Autodesk Fusion 360 part; units mm, degrees
sketch "Sketch1" plane through (0, 0, 0) normal (0, 0, 1) x (1, 0, 0)
  line L0 (69.2401, 97.5535) -> (12.2401, 97.5535)
  line L1 (12.2401, 97.5535) -> (12.2401, 48.4535)
  line L2 (52.8401, 84.1535) -> (28.6401, 84.1535)
  line L3 (59.3712, 82.4035) -> (64.1343, 79.6535)
  line L4 (64.1343, 79.6535) -> (69.2401, 79.6535)
  line L5 (69.2401, 79.6535) -> (69.2401, 97.5535)
  line L6 (22.109, 82.4035) -> (14.2401, 77.8603)
  line L7 (14.2401, 77.8603) -> (14.2401, 61.3991)
  line L8 (14.2401, 61.3991) -> (22.3734, 55.0972)
  line L9 (28.5401, 52.1228) -> (28.5401, 48.4535)
  line L10 (28.5401, 48.4535) -> (12.2401, 48.4535)
  arc A0 (59.3712, 82.4035) -> (52.8401, 84.1535) centre (56.3401, 84.1535) ccw
  arc A1 (28.6401, 84.1535) -> (22.109, 82.4035) centre (25.1401, 84.1535) ccw
  arc A2 (22.3734, 55.0972) -> (28.5401, 52.1228) centre (25.1401, 52.9535) ccw
  line L11 (14.2401, 50.4535) -> (14.2401, 58.869)
  line L12 (14.2401, 58.869) -> (19.6401, 54.6849)
  line L13 (19.6401, 54.6849) -> (14.2401, 50.4535)
  line L14 (14.2401, 86.1535) -> (22.9682, 95.5535)
  line L15 (22.9682, 95.5535) -> (14.2401, 95.5535)
  line L16 (14.2401, 95.5535) -> (14.2401, 86.1535)
  line L17 (26.3674, 95.5535) -> (32.3674, 86.1535)
  line L18 (32.3674, 86.1535) -> (38.3674, 95.5535)
  line L19 (38.3674, 95.5535) -> (26.3674, 95.5535)
  line L20 (49.1128, 86.1535) -> (55.1128, 95.5535)
  line L21 (55.1128, 95.5535) -> (43.1128, 95.5535)
  line L22 (43.1128, 95.5535) -> (49.1128, 86.1535)
  line L23 (34.7401, 86.1535) -> (46.7401, 86.1535)
  line L24 (46.7401, 86.1535) -> (40.7401, 95.5535)
  line L25 (40.7401, 95.5535) -> (34.7401, 86.1535)
  dimension "d1" = 7
  dimension "d2" = 7
  dimension "d3" = 31.2
  dimension "d10" = 7
  dimension "d11" = 150
  dimension "d12" = 150
  dimension "d13" = 127.769
  dimension "d14" = 12.9
  dimension "d15" = 12.9
  dimension "d16" = 31.2
  dimension "d17" = 4.5
  dimension "d18" = 13.4
  dimension "d19" = 12.9
  dimension "d21" = 4.5
  dimension "d23" = 2
  dimension "d24" = 5.5
  dimension "d25" = 2
  dimension "d26" = 2
  dimension "d27" = 2
  dimension "d35" = 2
  dimension "d36" = 2
  dimension "d37" = 2
  dimension "d38" = 2
  dimension "d39" = 2
  dimension "d40" = 2
  dimension "d41" = 2
  dimension "d42" = 2
  dimension "d43" = 2
  dimension "d44" = 2
  dimension "d45" = 12
  dimension "d46" = 15.6
  dimension "d47" = 2
  dimension "d74" = 90
  dimension "d77" = 3.4
extrude "Extrude1" add sketch "Sketch1" along normal blind 12.5
sketch "Sketch2" plane through (0, 97.5535, 0) normal (0, 1, 0) x (-1, 0, 0)
  line L0 (-69.2401, 0) -> (-12.2401, 0)
  line L1 (-12.2401, 0) -> (-12.2401, 12.5)
  line L2 (-12.2401, 12.5) -> (-69.2401, 12.5)
  line L3 (-69.2401, 12.5) -> (-69.2401, 0)
  point P0 (-60.2401, 4.5)
  dimension "d30" = 9
  dimension "d31" = 8
hole "Hole1" at (60.2401, 97.5535, 4.5) direction (0, -1, 0) diameter 5 depth 10 tip angle 118
fillet "Fillet2" radius 1 15 edges at (55.1128, 95.5535, 6.25) (43.1128, 95.5535, 6.25) (49.1128, 86.1535, 6.25) (46.7401, 86.1535, 6.25) (40.7401, 95.5535, 6.25) (34.7401, 86.1535, 6.25) (38.3674, 95.5535, 6.25) (32.3674, 86.1535, 6.25) (26.3674, 95.5535, 6.25) (22.9682, 95.5535, 6.25) (14.2401, 86.1535, 6.25) (14.2401, 95.5535, 6.25) (19.6401, 54.6849, 6.25) (14.2401, 58.869, 6.25) (14.2401, 50.4535, 6.25)
sketch "Sketch3" plane through (0, 0, 0) normal (0, 0, -1) x (1, 0, 0)
  line L0 (69.2401, -79.6535) -> (64.1343, -79.6535)
  line L1 (64.1343, -79.6535) -> (59.3712, -82.4035)
  arc A0 (52.8401, -84.1535) -> (59.3712, -82.4035) centre (56.3401, -84.1535) ccw
  line L2 (52.8401, -84.1535) -> (28.6401, -84.1535)
  arc A1 (22.109, -82.4035) -> (28.6401, -84.1535) centre (25.1401, -84.1535) ccw
  line L3 (22.109, -82.4035) -> (14.2401, -77.8603)
  line L4 (14.2401, -77.8603) -> (14.2401, -61.3991)
  line L5 (14.2401, -61.3991) -> (22.3734, -55.0972)
  arc A2 (28.5401, -52.1228) -> (22.3734, -55.0972) centre (25.1401, -52.9535) ccw
  line L6 (28.5401, -52.1228) -> (28.5401, -48.4535)
  line L7 (28.5401, -48.4535) -> (12.2401, -48.4535)
  line L8 (12.2401, -48.4535) -> (12.2401, -97.5535)
  line L9 (12.2401, -97.5535) -> (69.2401, -97.5535)
  line L10 (69.2401, -97.5535) -> (69.2401, -79.6535)
  arc A3 (27.3491, -94.0154) -> (28.1921, -95.5535) centre (28.1921, -94.5535) ccw
  line L11 (27.3491, -94.0154) -> (31.5245, -87.474)
  arc A4 (33.2103, -87.474) -> (31.5245, -87.474) centre (32.3674, -88.0121) ccw
  line L12 (33.2103, -87.474) -> (37.3857, -94.0154)
  arc A5 (36.5428, -95.5535) -> (37.3857, -94.0154) centre (36.5428, -94.5535) ccw
  line L13 (36.5428, -95.5535) -> (28.1921, -95.5535)
  arc A6 (14.2401, -56.8291) -> (15.8526, -57.6196) centre (15.2401, -56.8291) ccw
  line L14 (14.2401, -56.8291) -> (14.2401, -52.5075)
  arc A7 (15.8569, -51.7204) -> (14.2401, -52.5075) centre (15.2401, -52.5075) ccw
  line L15 (15.8569, -51.7204) -> (18.6299, -53.8933)
  arc A8 (18.6256, -55.4709) -> (18.6299, -53.8933) centre (18.0131, -54.6805) ccw
  line L16 (18.6256, -55.4709) -> (15.8526, -57.6196)
  arc A9 (15.9729, -88.0197) -> (14.2401, -88.7001) centre (15.2401, -88.7001) ccw
  line L17 (15.9729, -88.0197) -> (21.4079, -93.873)
  arc A10 (20.6751, -95.5535) -> (21.4079, -93.873) centre (20.6751, -94.5535) ccw
  line L18 (20.6751, -95.5535) -> (15.2401, -95.5535)
  arc A11 (14.2401, -94.5535) -> (15.2401, -95.5535) centre (15.2401, -94.5535) ccw
  line L19 (14.2401, -94.5535) -> (14.2401, -88.7001)
  arc A12 (49.9557, -87.474) -> (48.2699, -87.474) centre (49.1128, -88.0121) ccw
  line L20 (49.9557, -87.474) -> (54.1311, -94.0154)
  arc A13 (53.2882, -95.5535) -> (54.1311, -94.0154) centre (53.2882, -94.5535) ccw
  line L21 (53.2882, -95.5535) -> (44.9375, -95.5535)
  arc A14 (44.0945, -94.0154) -> (44.9375, -95.5535) centre (44.9375, -94.5535) ccw
  line L22 (44.0945, -94.0154) -> (48.2699, -87.474)
  arc A15 (36.5648, -86.1535) -> (35.7218, -87.6915) centre (36.5648, -87.1535) ccw
  line L23 (36.5648, -86.1535) -> (44.9155, -86.1535)
  arc A16 (45.7584, -87.6915) -> (44.9155, -86.1535) centre (44.9155, -87.1535) ccw
  line L24 (45.7584, -87.6915) -> (41.583, -94.2329)
  arc A17 (39.8972, -94.2329) -> (41.583, -94.2329) centre (40.7401, -93.6948) ccw
  line L25 (39.8972, -94.2329) -> (35.7218, -87.6915)
  line L26 (12.2401, -48.4535) -> (14.2401, -48.4535)
  line L27 (12.2401, -48.4535) -> (12.2401, -97.5535)
  line L28 (12.2401, -97.5535) -> (14.2401, -97.5535)
  line L29 (14.2401, -97.5535) -> (14.2401, -48.4535)
  dimension "d51" = 2
  dimension "d52" = 2
extrude "Extrude2" add sketch "Sketch3" along normal blind 7.5 contours L4 L7 L8 L9 L14 L19 L26 L27 L28 L29
sketch "Sketch4" plane through (12.2401, 0, 0) normal (-1, 0, 0) x (0, -1, 0)
  line L0 (-48.4535, -7.5) -> (-48.4535, 12.5)
  line L1 (-48.4535, 12.5) -> (-97.5535, 12.5)
  line L2 (-97.5535, 12.5) -> (-97.5535, -7.5)
  line L3 (-97.5535, -7.5) -> (-48.4535, -7.5)
  line L4 (-93.5535, -1.3) -> (-73.5535, -1.3)
  arc A0 (-73.5535, -3.7) -> (-73.5535, -1.3) centre (-73.5535, -2.5) ccw
  line L5 (-73.5535, -3.7) -> (-93.5535, -3.7)
  arc A1 (-93.5535, -1.3) -> (-93.5535, -3.7) centre (-93.5535, -2.5) ccw
  arc A2 (-93.5535, 8.8) -> (-93.5535, 6.4) centre (-93.5535, 7.6) ccw
  arc A3 (-73.5535, 6.4) -> (-73.5535, 8.8) centre (-73.5535, 7.6) ccw
  line L6 (-73.5535, 6.4) -> (-93.5535, 6.4)
  line L7 (-93.5535, 8.8) -> (-73.5535, 8.8)
  line L8 (-97.5535, 12.5) -> (-48.4535, 12.5)
  line L9 (-48.4535, 12.5) -> (-48.4535, 11.5)
  line L10 (-48.4535, 11.5) -> (-97.5535, 11.5)
  line L11 (-97.5535, 11.5) -> (-97.5535, 12.5)
  line L12 (-97.5535, -7.5) -> (-48.4535, -7.5)
  line L13 (-48.4535, -7.5) -> (-48.4535, -6.9)
  line L14 (-48.4535, -6.9) -> (-97.5535, -6.9)
  line L15 (-97.5535, -6.9) -> (-97.5535, -7.5)
  dimension "d55" = 2.4
  dimension "d56" = 20
  dimension "d59" = 2.4
  dimension "d60" = 20
  dimension "d61" = 7.7
  dimension "d63" = 4
  dimension "d64" = 4
  dimension "d65" = 3.7
  dimension "d69" = 1
  dimension "d79" = 0.6
extrude "Extrude3" cut sketch "Sketch4" against normal blind 3 contours L4 A0 L5 A1 | A2 A3 L6 L7
extrude "Extrude4" add sketch "Sketch4" along normal blind 1 contours L0 L2 L3 L12 L13 L14 L15 | L0 L1 L2 L8 L9 L10 L11
fillet "Fillet3" radius 2 3 edges at (11.2401, 97.5535, -7.2) (11.2401, 97.5535, 12) (12.2401, 97.5535, 2.3)
fillet "Fillet3" radius 2 3 edges at (69.2401, 97.5535, 6.25) (69.2401, 79.6535, 6.25) (64.1343, 79.6535, 6.25)
fillet "Fillet3" radius 0.3 1 edges at (28.5401, 52.1228, 6.25)
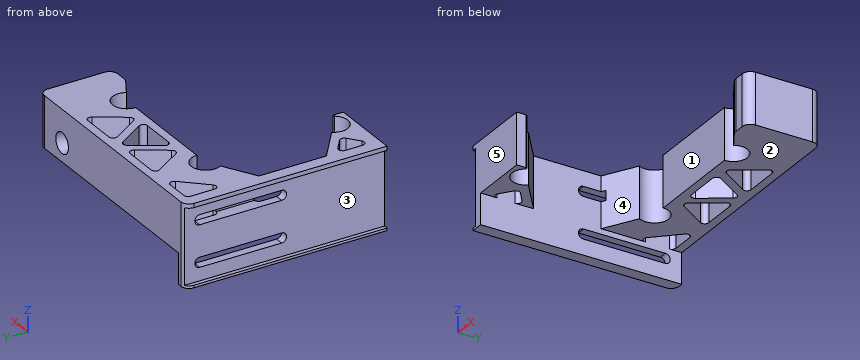
CAD build for the part. Positions are in the model's coordinates, mm. Face numbers are marked on the shaded views. A direction names the side the tool comes from. Give positions to 0.01 mm unless a question says otherwise; leave off trailing zeros. Write each loop counter-clockwise with the first axis right and the second up, starting at its lowest first coordinate (ties: lowest second). Pieces come first, ordered by that corner, then holes. Notation, with made-up numbers: (-28, -4.5) - (-20, -4.5) arc R23 ccw to (-20, 31.5) - close; hole circle Ø11 at (32.25, 44). An arc over 180 degrees is marked (long way). Put each result on its own line as item: value.
(1) Saw through at C-C (x = 24.5). List the corners of the cut face in (y, z).
Working result:
outline: (48.45, 0) - (49.51, 0) - (49.51, 12.5) - (48.45, 12.5) - close; (87.59, 0) - (97.55, 0) - (97.55, 12.5) - (87.59, 12.5) - close
(2) Saw through at A-A (y = 74.5). List the corners of the cut face in (x, z).
Working result:
outline: (11.24, -7.5) - (14.24, -7.5) - (14.24, -3.7) - (12.24, -3.7) - (12.24, -6.9) - (11.24, -6.9) - close; (11.24, 11.5) - (12.24, 11.5) - (12.24, 8.8) - (14.24, 8.8) - (14.24, 12.5) - (11.24, 12.5) - close; (12.24, -1.3) - (14.24, -1.3) - (14.24, 6.4) - (12.24, 6.4) - close
(3) Drop flat-ended pins along their axis: pin 1 Ø6 at (y, z) = (59, 6) entering from +X; pin 2 Ø6.5 at (x, z) = (49.5, 7) entering from -Y; pin 3 Ø11 at (x, y) = (25.14, 84.15) entering from -Z. Give the stop position or say it passes through.
Working result:
pin 1: x = 21.21
pin 2: y = 84.15
pin 3: z = 0
(4) Wall check: L1, parallel to X at y = 90, z = 4.5; L2, parallel to X at y = 94.25, z = 4.5; L3, parallel to X at y = 70, z = 5.75. Give the ranges that are in metal, low to high.
Working result:
L1: 12.24 to 14.24, 17.81 to 29.91, 34.82 to 37.2, 44.28 to 46.66, 51.57 to 57.74, 62.74 to 69.24
L2: 12.24 to 14.24, 21.63 to 27.24, 37.5 to 39.91, 41.57 to 43.98, 54.24 to 57.74, 62.74 to 69.24
L3: 12.24 to 14.24
(5) Saw through at D-D (z = 10.75). Count the separate pieces of the cut face and the enclosed holes in it, then the cut area to 3 significant figures.
Working result:
separate pieces: 1
enclosed holes: 5
area: 728 mm^2
(6) Tool access for the marked faces 4 and 5: list every direction of +Z, -Z, +X, -X, +Y, -Y with a clear straight run to the whole face (end or side of a thin tool).
Working result:
face 4: +Z, -Z
face 5: +Z, -Z, +X, -X, -Y
(7) Pull direction X, two halves, no side cores. Call the marked faces 1, 2 and 3: released by +X, released by -X, zero draft, split by the parting line, or undercut.
Working result:
face 1: undercut
face 2: zero draft
face 3: released by -X
(8) Saw through at B-B (y = 68). List the corners of the cut face in (x, z), then the cut area to 3 significant figures.
Working result:
outline: (11.24, -7.5) - (14.24, -7.5) - (14.24, 12.5) - (11.24, 12.5) - (11.24, 11.5) - (12.24, 11.5) - (12.24, -6.9) - (11.24, -6.9) - close
area: 41.6 mm^2
